Here's how the part is built. I have some questions about the finished solid (model axes, mm). Face numbers are marked on the shaded views. A direction names the side the tool comes from. Round coordinates to 2 decimals unless told otherwise and drop trailing zeros. Write each loop counter-clockwise with the first axis right and the second up, starting at its lowest first coordinate (ties: lowest second). Pieces come first, ordered by that corner, then holes. Notation, with made-up numbers: (42.25, 68.25) -> (79.25, 68.25) arc R32 ccw to (79.25, 96.25) -> close; hole circle Ø2 at (35.5, 72). An arc over 180 degrees is marked (long way). Put each result on its own line as item: value. Start each with the question number.
1. I need wall thicknesses on probe 1 along Z at (x, y) = (0, -13); probe 2 along X at (y, z) = (-12.05, 24); probe 3 along Y at (x, z) = (-6.5, 20). Which ranges of each line are inside material? Lowest first, please. Write a range as from..to.
2. We'd pull the mould along X, two halves only. Please class the marked faces 4, 5 and 6: +X half, -X half, draft (parallel to the pull), parting line (faces both ways), or undercut.
3. Which directions (+Z, -Z, +X, -X, +Y, -Y) give clear straight access to the entire face, cutting with the end or side of a thin tool? Please do the marked faces 1, 2 and 3.
4. For pin 1 (1.6 mm diameter, centred on y = -17, z = 28.5, fed in from +X); pin 2 (6.5 mm diameter, centred on x = 0, z = 24, fed in from -Y); pin 3 (0.8 mm diameter, centred on y = -17, z = 29.5, fed in from -X), each with a flat end and sliding along its axis, tell me the tip position at first contact or that it passes through.
5. Suppose I cut it at B-B (y = 6). Please give me the cut outline in (x, z).
6. Suppose I cut it at A-A (x = 0). Count the separate pieces of the cut face and the enclosed holes in it, then the cut area to 3 significant figures.
7. Suppose I cut it at C-C (y = -15). Please give me the cut outline in (x, z), then the cut area to 3 significant figures.
8. Suppose I cut it at D-D (x = -21). Please give me the cut outline in (y, z).
Autodesk Inventor part; units mm, degrees
ref_plane "YZ Plane" through (0, 0, 0) normal (1, 0, 0) x (0, 1, 0)
ref_plane "XZ Plane" through (0, 0, 0) normal (0, 1, 0) x (-1, 0, 0)
ref_plane "XY Plane" through (0, 0, 0) normal (0, 0, 1) x (1, 0, 0)
sketch "Sketch1" plane through (0, 0, 0) normal (0, 0, 1) x (1, 0, 0)
  line L0 (-12.2491, 0) -> (12.2491, 0)
  line L1 (0, 10.917) -> (0, -10.917)
  line L2 (-30, -10) -> (-30, -16)
  line L3 (-30, -16) -> (16, -16)
  line L4 (-30, -10) -> (10, -10)
  line L5 (10, -10) -> (10, 10)
  line L6 (10, 10) -> (-30, 10)
  line L7 (-30, 10) -> (-30, 16)
  line L8 (-30, 16) -> (16, 16)
  line L9 (16, 16) -> (16, -16)
  point P0 (0, 0)
  point P1 (0, 0)
  dimension "d0" = 10
  dimension "d1" = 10
  dimension "d2" = 10
  dimension "d3" = 30
  dimension "d4" = 6
  dimension "d5" = 6
  dimension "d6" = 40
  dimension "d7" = 6
extrude "Extrusion1" add sketch "Sketch1" along normal blind 30 contours L5 L6 L7 L8 L9 L3 L2 L4
sketch "Sketch2" plane through (-30, -16, 0) normal (0, -1, 0) x (1, 0, 0)
  line L0 (40, 30) -> (0, 30)
  line L1 (27, 30) -> (27, 0)
  line L2 (0, 0) -> (0, 30)
  line L3 (33, 30) -> (33, 0)
  line L4 (40, 0) -> (0, 0)
  line L5 (27, 30) -> (33, 30)
  line L6 (33, 0) -> (27, 0)
  line L7 (46, 0) -> (46, 30)
  line L8 (40, 0) -> (40, 30)
  point P0 (30, 0)
  dimension "d37" = 13
  dimension "d38" = 7
extrude "Extrusion2" add sketch "Sketch2" along normal blind 1.5 contours L3 L4 L1 L0
sketch "Sketch3" plane through (-30, -17.5, 0) normal (0, -1, 0) x (1, 0, 0)
  line L0 (27, 0) -> (33, 0)
  line L1 (27, 30) -> (27, 0)
  line L2 (27, 15) -> (13, 15)
  line L3 (33, 0) -> (33, 30)
  point P0 (30, 0)
  point P1 (30, 6)
  point P2 (30, 24)
  dimension "d14" = 6
  dimension "d36" = 3
hole "Hole1" at (0, -17.5, 6) at (0, -17.5, 24) direction (0, 1, 0) diameter 5.5 end up to surface counterbore diameter 10 counterbore depth 1.5
sketch "Sketch4" plane through (-30, 16, 0) normal (0, 1, 0) x (1, 0, 0)
  arc A0 (7, -11.75) -> (7, -18.25) centre (7, -15) ccw
  line L0 (0, 0) -> (0, -30)
  line L1 (46, 0) -> (0, 0)
  arc A1 (34, -18.25) -> (34, -11.75) centre (34, -15) ccw
  line L2 (46, -30) -> (0, -30)
  line L3 (34, -11.75) -> (7, -11.75)
  line L4 (34, -18.25) -> (7, -18.25)
  point P0 (30, 0)
  dimension "d22" = 6.5
  dimension "d23" = 7
  dimension "d24" = 15
  dimension "d25" = 6.5
  dimension "d26" = 34
  dimension "d27" = 15
extrude "Extrusion3" cut sketch "Sketch4" against normal up to surface (6 mm away)
sketch "Sketch5" plane through (-30, -16, 0) normal (-1, 0, 0) x (0, 0, 1)
  line L0 (0, 0) -> (0, 32)
  line L1 (30, 6) -> (30, 0)
  line L2 (0, 32) -> (30, 32)
  line L3 (30, 32) -> (30, 0)
  line L4 (30, 0) -> (0, 0)
  line L5 (0, 0) -> (0, 32)
  point P0 (0, 16)
extrude "Extrusion4" add sketch "Sketch5" along normal blind 6
fillet "Fillet3" radius 2 8 edges at (16, 0, 30) (-10, 16, 30) (-36, 16, 15) (-36, 0, 30) (-36, 0, 0) (-10, 16, 0) (16, 16, 15) (16, 0, 0)
properties part number "Estrutura - Suporte Mesa"
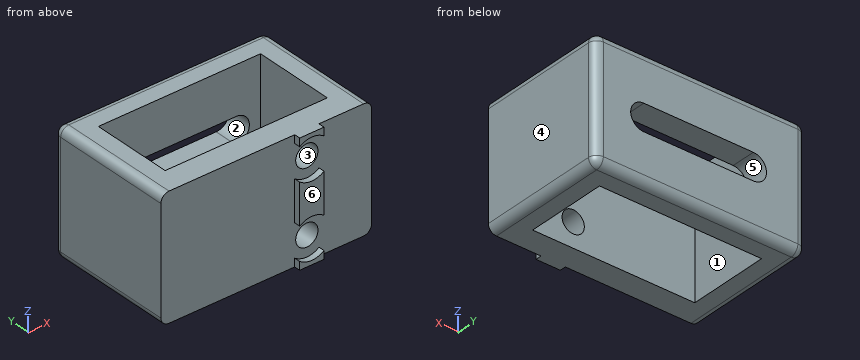
Verdict:
1. probe 1: z = 0..3.25, 8.75..21.25, 26.75..30
1. probe 2: x = -36..-2.75, 2.75..16
1. probe 3: y = -16..-10, 10..16
2. face 4: +X half
2. face 5: undercut
2. face 6: draft
3. face 1: +Z, -Z
3. face 2: +Y
3. face 3: -Y
4. pin 1: stops at x = 3
4. pin 2: stops at y = -16
4. pin 3: stops at x = -3
5. outline: (-36, 2) arc R2 ccw to (-34, 0) -> (-30, 0) -> (-30, 30) -> (-34, 30) arc R2 ccw to (-36, 28) -> close; (10, 0) -> (14, 0) arc R2 ccw to (16, 2) -> (16, 28) arc R2 ccw to (14, 30) -> (10, 30) -> close
6. separate pieces: 5
6. enclosed holes: 0
6. area: 268 mm^2
7. outline: (-36, 2) arc R2 ccw to (-34, 0) -> (14, 0) arc R2 ccw to (16, 2) -> (16, 28) arc R2 ccw to (14, 30) -> (-34, 30) arc R2 ccw to (-36, 28) -> close; hole circle Ø5.5 at (0, 6); hole circle Ø5.5 at (0, 24)
7. area: 1,510 mm^2
8. outline: (-16, 0) -> (-10, 0) -> (-10, 30) -> (-16, 30) -> close; (10, 0) -> (14, 0) arc R2 ccw to (16, 2) -> (16, 11.75) -> (10, 11.75) -> close; (10, 18.25) -> (16, 18.25) -> (16, 28) arc R2 ccw to (14, 30) -> (10, 30) -> close
